Geometry check sheet. Reference: the model listing, model coordinates, mm. Face numbers are marked on the shaded views. A direction names the side the tool comes from. Give positions to 0.01 mm unless a question says otherwise; leave off trailing zeros. Loops run counter-clockwise (first coordinate to the right, second up) from the corner with the lowest first, then second, coordinate; pieces in that order, holes last. Notation, with made-up numbers: (-5, 11.25) -> (44, 11.25) arc R18 cw to (44, 45.25) -> close; hole circle Ø4 at (-21.5, 69.25). An arc over 180 degrees is marked (long way). One line per item, written item: value. Start each with the question number.
(1) Scan lines: line 1 along X through (y, z) = (-10, 1.25); line 2 along Y through (x, z) = (0, 2.6); line 3 along X through (y, z) = (-8.5, 3.5). Record each from-to range of solid material in increasing order. Write a range as from..to.
(2) Sectioned sample at A-A, the plane y = -1.5. Record the cut outline in (x, z).
(3) Tool access check on the marked faces 1, 2, 3 and 4. Record the directions out of +Z, -Z, +X, -X, +Y, -Y that give a thin tool (end or side, any length) a straight path to the whole face; none if there is none.
(4) Sectioned sample at D-D, the plane y = 2.25. Record the cut outline in (x, z).
(5) Draft check along X on the marked faces 5, 6, 7 and 8. Enter one of: pulls with the +X half, pulls with the -X half, needs draft (parallel to the pull), parting line crosses it, or undercut.
(6) Sectioned sample at C-C, the plane x = 0. Record the cut outline in (y, z).
(7) Gauge pin test, flat ends, axial feed: pin 1 Ø0.5 at (y, z) = (-9, 2.5) entering from +X; pin 2 Ø2 at (x, z) = (-1, 2) entering from -Y; pin 3 Ø1.5 at (x, z) = (-0.5, 3.5) entering from +Y. Record the tip position at first contact, or that the pin passes through.
(8) Sectioned sample at B-B, the plane z = 3.75. Record the cut outline in (x, y), then the cut area to 3 significant figures.
from build123d import *

# Parameters (mm, degrees)
PAD_DEPTH = 4


with BuildPart() as part:
    # Sketch → Pad (new body)
    with BuildSketch(Plane.XY):
        with BuildLine():
            Line((-6.25, -6.24398), (-6.25, -11.24398))
            Line((-6.25, -11.24398), (-3.25, -11.24398))
            Line((-3.25, -11.24398), (-3.25, -9.24398))
            Line((-3.25, -9.24398), (-4.25, -9.24398))
            Line((-4.25, -9.24398), (-4.25, -8.24398))
            Line((-4.25, -8.24398), (4.25, -8.24398))
            Line((4.25, -8.24398), (4.25, -9.24398))
            Line((4.25, -9.24398), (3.25, -9.24398))
            Line((3.25, -9.24398), (3.25, -11.24398))
            Line((3.25, -11.24398), (6.25, -11.24398))
            Line((6.25, -11.24398), (6.25, -6.24398))
            ThreePointArc((6.25, -6.24398), (8.424703, 0.213043), (5.133293, 6.178704))
            Line((4.277996, 3.733721), (5.133293, 6.178704))
            ThreePointArc((-4.277996, 3.733721), (0, -6.594275), (4.277996, 3.733721))
            Line((-4.277996, 3.733721), (-5.133293, 6.178704))
            ThreePointArc((-5.133293, 6.178704), (-8.424703, 0.213043), (-6.25, -6.24398))
        make_face()
    extrude(amount=PAD_DEPTH)


solid = part.part
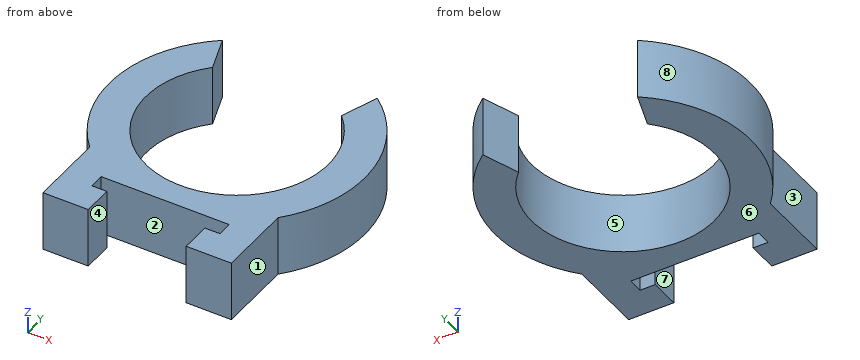
Calculated:
1. line 1: x = -6.25..-3.25, 3.25..6.25
1. line 2: y = -8.24..-6.59
1. line 3: x = -6.25..-4.25, 4.25..6.25
2. outline: (-8.4, 0) -> (-5.97, 0) -> (-5.97, 4) -> (-8.4, 4) -> close; (5.97, 0) -> (8.4, 0) -> (8.4, 4) -> (5.97, 4) -> close
3. face 1: +Z, -Z, +X, -Y
3. face 2: +Z, -Z
3. face 3: +Z, -Z, -X, -Y
3. face 4: +Z, -Z, -Y
4. outline: (-7.98, 0) -> (-5.37, 0) -> (-5.37, 4) -> (-7.98, 4) -> close; (5.37, 0) -> (7.98, 0) -> (7.98, 4) -> (5.37, 4) -> close
5. face 5: undercut
5. face 6: needs draft
5. face 7: undercut
5. face 8: pulls with the -X half
6. outline: (-8.24, 0) -> (-6.59, 0) -> (-6.59, 4) -> (-8.24, 4) -> close
7. pin 1: stops at x = 6.25
7. pin 2: stops at y = -8.24
7. pin 3: stops at y = -6.46
8. outline: (-6.25, -11.24) -> (-3.25, -11.24) -> (-3.25, -9.24) -> (-4.25, -9.24) -> (-4.25, -8.24) -> (4.25, -8.24) -> (4.25, -9.24) -> (3.25, -9.24) -> (3.25, -11.24) -> (6.25, -11.24) -> (6.25, -6.24) arc R8.46 ccw to (5.13, 6.18) -> (4.28, 3.73) arc R6.05 cw (long way) to (-4.28, 3.73) -> (-5.13, 6.18) arc R8.46 ccw to (-6.25, -6.24) -> close
8. area: 102 mm2
